```python
from build123d import *

# Parameters (mm, degrees)
SKETCH1_W           = 25
SKETCH1_H           = 15
SKETCH1_R           = 0.85
BOSS_EXTRUDE1_DEPTH = 1
SKETCH2_W           = 26
SKETCH2_H           = 15
SKETCH2_R           = 0.85
BOSS_EXTRUDE2_DEPTH = 1


with BuildPart() as part:
    # Sketch1 → Boss-Extrude1 (new body)
    with BuildSketch(Plane.XY):
        Rectangle(SKETCH1_W, SKETCH1_H)
        with Locations((7.5, 0)):
            Circle(SKETCH1_R, mode=Mode.SUBTRACT)
    extrude(amount=BOSS_EXTRUDE1_DEPTH)

    # Sketch2 → Boss-Extrude2 (add)
    with BuildSketch(Plane.ZY.offset(12.5)):
        with Locations((-12, 0)):
            Rectangle(SKETCH2_W, SKETCH2_H)
        with Locations((-20, 0)):
            Circle(SKETCH2_R, mode=Mode.SUBTRACT)
    extrude(amount=BOSS_EXTRUDE2_DEPTH)


solid = part.part
```
Read the model definition and answer for the solid it produces. Units are mm, in the model's axes. A direction names the side the tool comes from. Give positions to 0.01 mm unless a question says otherwise; leave off trailing zeros. Write each loop counter-clockwise with the first axis right and the second up, starting at its lowest first coordinate (ties: lowest second). Pieces come first, ordered by that corner, then holes. Notation, with made-up numbers: (15, -17) - (27, -17) arc R23 cw to (27, 13) - close; hole circle Ø6 at (-21.5, 60). An arc over 180 degrees is marked (long way). Write item = value, one per line. Start each with the question number.
Item 1: Find section A-A (y = 0). Give the vertices of the cut face in (x, z).
Item 2: Find section C-C (x = 7.5). Give the vertices of the cut face in (y, z), then the cut area to 3 significant figures.
Item 3: Find section D-D (y = -5.75). Give the vertices of the cut face in (x, z), then the cut area to 3 significant figures.
Item 4: Each of these flat-tipped pins is pushed along its axis until it touches: P1, Ø5, axis at x = -6, y = -5.5, coming from the -Z side; P2, Ø1.5, axis at y = 0.5, z = -8.5, coming from the +X side. Where does it stop, or does it pass through?
Item 5: Find section B-B (z = -20). Give the vertices of the cut face in (x, y), then the cut area to 3 significant figures.
Item 6: The mould has two halves that part along Y. Classify faces 1 (the flat face through (-13, 7.5, -6)), 2 (the cylindrical face through (-12.99, -0.52, -20.67)), 3 (the flat face through (12.5, -0.1, 0.5)): +Y half, -Y half, draft (parallel to the pull), parting line (faces both ways), or undercut.
Item 7: A tool of negligible diameter and unlimited length cuts with its end or side. For faces 4 (the flat face through (-12.5, 0, -13)), 5 (the flat face through (0, 0, 1)), from which of +Z, -Z, +X, -X, +Y, -Y can it reach the whole face along a straight path? Write none if from no direction.
Item 8: Find the intervals of material crossed by probe 1 along Y at (x, z) = (-13.2, -20); probe 2 along X at (y, z) = (3, -17.75); probe 3 along Z at (x, y) = (-11.25, 4.5), in increasing order. Write a range as [from, to].
Response:
q1.outline = (-13.5, -25) - (-12.5, -25) - (-12.5, -20.85) - (-13.5, -20.85) - close; (-13.5, -19.15) - (-12.5, -19.15) - (-12.5, 0) - (6.65, 0) - (6.65, 1) - (-13.5, 1) - close; (8.35, 0) - (12.5, 0) - (12.5, 1) - (8.35, 1) - close
q2.outline = (-7.5, 0) - (-0.85, 0) - (-0.85, 1) - (-7.5, 1) - close; (0.85, 0) - (7.5, 0) - (7.5, 1) - (0.85, 1) - close
q2.area = 13.3 mm²
q3.outline = (-13.5, -25) - (-12.5, -25) - (-12.5, 0) - (12.5, 0) - (12.5, 1) - (-13.5, 1) - close
q3.area = 51.0 mm²
q4.P1 = 0
q4.P2 = -12.5
q5.outline = (-13.5, -7.5) - (-12.5, -7.5) - (-12.5, -0.85) - (-13.5, -0.85) - close; (-13.5, 0.85) - (-12.5, 0.85) - (-12.5, 7.5) - (-13.5, 7.5) - close
q5.area = 13.3 mm²
q6.face_1 = +Y half
q6.face_2 = undercut
q6.face_3 = draft
q7.face_4 = -Z, +X, +Y, -Y
q7.face_5 = +Z, +X, -X, +Y, -Y
q8.probe_1 = [-7.5, -0.85], [0.85, 7.5]
q8.probe_2 = [-13.5, -12.5]
q8.probe_3 = [0, 1]
